from build123d import *

# Parameters (mm, degrees)
F0_W     = 70
F0_H     = 70
F1_DEPTH = 1
F2_W     = 70
F2_H     = 70
F2_W_2   = 68
F2_H_2   = 68
F3_DEPTH = 9
F4_W     = 15
F4_H     = 5
F5_DEPTH = 1
F6_R     = 1
F7_DEPTH = 4


with BuildPart() as f1:
    # F0 (on Top) → F1 (new body)
    with BuildSketch(Plane.XY):
        with Locations((-35, 35)):
            Rectangle(F0_W, F0_H)
    extrude(amount=F1_DEPTH)

    # F2 (on face) → F3 (join)
    with BuildSketch(Plane.XY.offset(1)):
        with Locations((-35, 35)):
            Rectangle(F2_W, F2_H)
        with Locations((-35, 35)):
            Rectangle(F2_W_2, F2_H_2, mode=Mode.SUBTRACT)
    extrude(amount=F3_DEPTH)

    # F4 (on face) → F5 (cut)
    with BuildSketch(Plane.XZ):
        with Locations((-35, 3.6)):
            Rectangle(F4_W, F4_H)
    extrude(amount=-F5_DEPTH, mode=Mode.SUBTRACT)

    # F6 (on face) → F7 (join)
    with BuildSketch(Plane.XY.offset(1)):
        with Locations((-63, 38)):
            Circle(F6_R)
        with Locations((-7, 38)):
            Circle(F6_R)
        with Locations((-7, 11)):
            Circle(F6_R)
        with Locations((-63, 11)):
            Circle(F6_R)
    extrude(amount=F7_DEPTH)


solid = f1.part
Geometry check sheet. Reference: the model listing, model coordinates, mm. A direction names the side the tool comes from. Give positions to 0.01 mm unless a question says otherwise; leave off trailing zeros. Write each loop counter-clockwise with the first axis right and the second up, starting at its lowest first coordinate (ties: lowest second). Pieces come first, ordered by that corner, then holes.
1) Thickness scan on line 1 (X direction, y = 64.5, z = 8.5); line 2 (Y direction, x = -19.5, z = 7.25); line 3 (Z direction, x = -53, y = 21). Record the ranges inside material, lowest first.
Values follow:
line 1: x = -70 to -69, -1 to 0
line 2: y = 0 to 1, 69 to 70
line 3: z = 0 to 1
2) Set-up check for faces 1 (the face through (-35, 35, 0)), 2 (the face through (-35, 69, 5)): record each of +Z, -Z, +X, -X, +Y, -Y from which the full face is reachable in a straight line by a thin tool's end or side.
Values follow:
face 1: -Z, +X, -X, +Y, -Y
face 2: +Z
3) Release check for a two-part mould opening along Y. For faces 3 (the face through (-35, 70, 5)), 4 (the face through (-7, 11, 5)), 5 (the face through (-70, 35, 5)) record: released by +Y, released by -Y, zero draft, split by the parting line, or undercut.
Values follow:
face 3: released by +Y
face 4: undercut
face 5: zero draft
4) Cross-section at A-A (z = 7). Record the boundary of the cut face in (x, y), plus the area to 3 significant figures.
Values follow:
outline: (-70, 0) - (0, 0) - (0, 70) - (-70, 70) - close; hole (-69, 1) - (-1, 1) - (-1, 69) - (-69, 69) - close
area: 276 mm2
5) Cross-section at D-D (x = -63). Record the boundary of the cut face in (y, z).
Values follow:
outline: (0, 0) - (70, 0) - (70, 10) - (69, 10) - (69, 1) - (39, 1) - (39, 5) - (37, 5) - (37, 1) - (12, 1) - (12, 5) - (10, 5) - (10, 1) - (1, 1) - (1, 10) - (0, 10) - close
6) Go/stop test with flat-tipped pins: pin 1 Ø2.5 at (x, z) = (-34.5, 4.5) entering from -Y; pin 2 Ø1 at (x, y) = (-12.5, 28.5) entering from +Z; pin 3 Ø1 at (x, y) = (-7, 11.5) entering from +Z. Record where each tip stops, or that it passes through.
Values follow:
pin 1: stops at y = 69
pin 2: stops at z = 1
pin 3: stops at z = 5
7) Cross-section at C-C (z = 3.5). Record the boundary of the cut face in (x, y), plus the area to 3 significant figures.
Values follow:
outline: (-70, 0) - (-42.5, 0) - (-42.5, 1) - (-69, 1) - (-69, 69) - (-1, 69) - (-1, 1) - (-27.5, 1) - (-27.5, 0) - (0, 0) - (0, 70) - (-70, 70) - close; circle Ø2 at (-63, 11); circle Ø2 at (-63, 38); circle Ø2 at (-7, 11); circle Ø2 at (-7, 38)
area: 274 mm2
8) Cross-section at B-B (y = 38). Record the boundary of the cut face in (x, z).
Values follow:
outline: (-70, 0) - (0, 0) - (0, 10) - (-1, 10) - (-1, 1) - (-6, 1) - (-6, 5) - (-8, 5) - (-8, 1) - (-62, 1) - (-62, 5) - (-64, 5) - (-64, 1) - (-69, 1) - (-69, 10) - (-70, 10) - close
